For this review, take the finished solid that the model builds, in its own axes (mm). Coordinates: 2 decimals unless noted, no trailing zeros. Write each loop counter-clockwise with the first axis right and the second up, starting at its lowest first coordinate (ties: lowest second). Pieces come first, ordered by that corner, then holes.
```python
from build123d import *

# Parameters (mm, degrees)
BOSS_EXTRUDE1_DEPTH = 3.175
SKETCH3_R           = 2.25
SKETCH3_R_2         = 1.5875
SKETCH3_W           = 13
SKETCH3_H           = 24
CUT_EXTRUDE1_DEPTH  = 7.35


with BuildPart() as part:
    # Sketch1 → Boss-Extrude1 (new body, symmetric)
    with BuildSketch(Plane.XY):
        Polygon((60, 0), (-60, 0), (-60, 80), (-15, 130), (15, 130), (60, 80), align=None)
    extrude(amount=BOSS_EXTRUDE1_DEPTH, both=True)

    # Sketch3 → Cut-Extrude1 (cut, through all)
    with BuildSketch(Plane.XY.offset(3.175)):
        with Locations((-52.9, 13)):
            Circle(SKETCH3_R)
        with Locations((-27.5, 13)):
            Circle(SKETCH3_R)
        with Locations((27.5, 13)):
            Circle(SKETCH3_R)
        with Locations((52.9, 13)):
            Circle(SKETCH3_R)
        with Locations((-50, 80)):
            Circle(SKETCH3_R_2)
        with Locations((-50, 51.425)):
            Circle(SKETCH3_R_2)
        with Locations((50, 51.425)):
            Circle(SKETCH3_R_2)
        with Locations((50, 80)):
            Circle(SKETCH3_R_2)
        with Locations((0, 110)):
            Rectangle(SKETCH3_W, SKETCH3_H)
    extrude(amount=-CUT_EXTRUDE1_DEPTH, mode=Mode.SUBTRACT)


solid = part.part
```
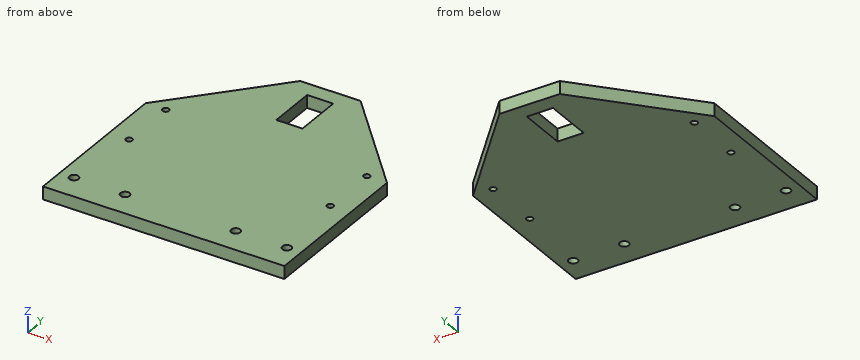
1) Consider section B-B (x = 2.5). Give the boundary of the cut face in (y, z) (3 decimals).
2) Consider section D-D (z = -1.5). Count the separate pieces of the cut face and the enclosed holes in it, then the cut area to 3 significant figures.
3) Clearance check with flat-ended pins moving along their axes: P1, Ø5, axis at x = 50, y = 51.425, coming from the -Z side (3 decimals); P2, Ø3, axis at x = 34, z = -2.5, coming from the +Y side; P3, Ø1.9, axis at y = 110.5, z = -1.5, coming from the -X side (3 decimals). State where each tip first meets the part, or that it passes through.
4) Consider section C-C (y = 118.5). Give the boundary of the cut face in (x, z) (3 decimals).
5) Consider section A-A (y = 13). Give the boundary of the cut face in (x, z) (3 decimals).
6) For L1, parallel to X at y = 80, z = -1.5; L2, parallel to Y at x = -3, z = 0.75; L3, parallel to Y at x = 50, z = 1, list the stretches that pass through material, from the lowest coordinate up.
Results:
1. outline: (0, -3.175) - (98, -3.175) - (98, 3.175) - (0, 3.175) - close; (122, -3.175) - (130, -3.175) - (130, 3.175) - (122, 3.175) - close
2. separate pieces: 1
2. enclosed holes: 9
2. area: 12,900 mm2
3. P1: stops at z = -3.175
3. P2: stops at y = 110.56
3. P3: stops at x = -33.405
4. outline: (-25.35, -3.175) - (-6.5, -3.175) - (-6.5, 3.175) - (-25.35, 3.175) - close; (6.5, -3.175) - (25.35, -3.175) - (25.35, 3.175) - (6.5, 3.175) - close
5. outline: (-60, -3.175) - (-55.15, -3.175) - (-55.15, 3.175) - (-60, 3.175) - close; (-50.65, -3.175) - (-29.75, -3.175) - (-29.75, 3.175) - (-50.65, 3.175) - close; (-25.25, -3.175) - (25.25, -3.175) - (25.25, 3.175) - (-25.25, 3.175) - close; (29.75, -3.175) - (50.65, -3.175) - (50.65, 3.175) - (29.75, 3.175) - close; (55.15, -3.175) - (60, -3.175) - (60, 3.175) - (55.15, 3.175) - close
6. L1: x = -60 to -51.59, -48.41 to 48.41, 51.59 to 60
6. L2: y = 0 to 98, 122 to 130
6. L3: y = 0 to 49.84, 53.01 to 78.41, 81.59 to 91.11
